from build123d import *

# Parameters (mm, degrees)
CROQUIS1_W              = 20
CROQUIS1_H              = 45
SALIENTE_EXTRUIR1_DEPTH = 228.2
CROQUIS5_W              = 17.6
CROQUIS5_H              = 42.6
CORTAR_EXTRUIR3_DEPTH   = 228.2
CROQUIS6_R              = 1.5
CORTAR_EXTRUIR4_DEPTH   = 30


with BuildPart() as part:
    # Croquis1 → Saliente-Extruir1 (new body)
    with BuildSketch(Plane.XY):
        Rectangle(CROQUIS1_W, CROQUIS1_H)
    extrude(amount=SALIENTE_EXTRUIR1_DEPTH)

    # Croquis5 → Cortar-Extruir3 (cut)
    with BuildSketch(Plane(origin=(0, 0, 0), x_dir=(-1, 0, 0), z_dir=(0, 0, -1))):
        Rectangle(CROQUIS5_W, CROQUIS5_H)
    extrude(amount=-CORTAR_EXTRUIR3_DEPTH, mode=Mode.SUBTRACT)

    # Croquis6 → Cortar-Extruir4 (cut)
    with BuildSketch(Plane(origin=(10, 0, 0), x_dir=(0, 0, -1), z_dir=(1, 0, 0))):
        with Locations((-210.2, -12)):
            Circle(CROQUIS6_R)
        with Locations((-210.2, 12)):
            Circle(CROQUIS6_R)
        with Locations((-18, 12)):
            Circle(CROQUIS6_R)
        with Locations((-18, -12)):
            Circle(CROQUIS6_R)
    extrude(amount=-CORTAR_EXTRUIR4_DEPTH, mode=Mode.SUBTRACT)


solid = part.part
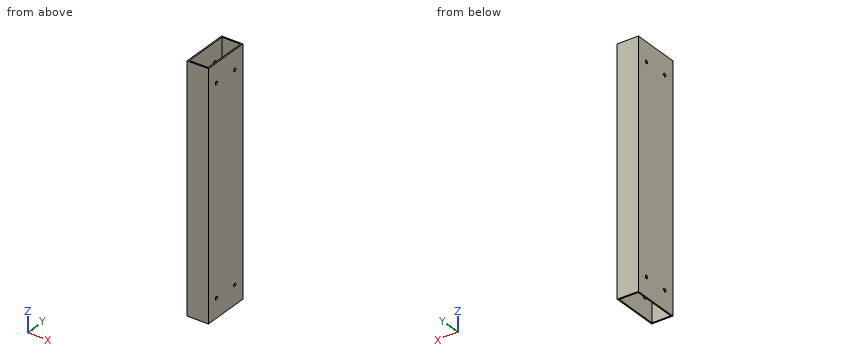
Can you work these out from the model? Positions are in its coordinate system, mm. Give positions to 0.01 mm unless a question says otherwise; leave off trailing zeros. Order: outer loops, then holes, each group sorted by start corner. A loop starts at its lowest first (then second) coordinate and runs counter-clockwise, first axis right, second up. Notation, with made-up numbers: M 35.5,58 L 47.5,58 A17 ccw 47.5,72 Z; hole C 77.25,4.5 d7. An arc over 180 degrees is marked long. Use a Markdown table: item, result. Add a question column.
Item 1: Suppose I cut it at A-A (x = 4.75). List the corners of the cut face in (y, z) for me.
Item 2: Will this pin go through, and if not, where does the flat tip stop? pin 1 (4 mm diameter, centred on x = -4.5, y = 17.5, fed in from +Z).
Item 3: Suppose I cut it at B-B (z = 141). List the corners of the cut face in (x, y) for me, then the cut area to 3 significant figures.
Item 4: If I drill on L1, parallel to Y at x = -9.1, z = 210.2; L2, parallel to X at y = -9.5, z = 70; L3, parallel to Y at x = -4, z = 88, over which ranges is the centre line in solid material (lowest first)? Write a range as [from, to].
Item 5: Suppose I cut it at C-C (y = -17.5). List the corners of the cut face in (x, z) for me, then the cut area to 3 significant figures.
Answer sheet:
| question | item | result |
|---|---|---|
| 1 | outline | M -22.5,0 L -21.3,0 L -21.3,228.2 L -22.5,228.2 Z; M 21.3,0 L 22.5,0 L 22.5,228.2 L 21.3,228.2 Z |
| 2 | pin 1 | passes through |
| 3 | outline | M -10,-22.5 L 10,-22.5 L 10,22.5 L -10,22.5 Z; hole M -8.8,-21.3 L 8.8,-21.3 L 8.8,21.3 L -8.8,21.3 Z |
| 3 | area | 150 mm² |
| 4 | L1 | y = [-22.5, -13.5], [-10.5, 10.5], [13.5, 22.5] |
| 4 | L2 | x = [-10, -8.8], [8.8, 10] |
| 4 | L3 | y = [-22.5, -21.3], [21.3, 22.5] |
| 5 | outline | M -10,0 L -8.8,0 L -8.8,228.2 L -10,228.2 Z; M 8.8,0 L 10,0 L 10,228.2 L 8.8,228.2 Z |
| 5 | area | 548 mm² |
